Autodesk Inventor part; units mm, degrees
ref_plane "YZ Plane" through (0, 0, 0) normal (1, 0, 0) x (0, 1, 0)
ref_plane "XZ Plane" through (0, 0, 0) normal (0, 1, 0) x (-1, 0, 0)
ref_plane "XY Plane" through (0, 0, 0) normal (0, 0, 1) x (1, 0, 0)
sketch "Sketch1" plane through (0, 0, 0) normal (0, 1, 0) x (-1, 0, 0)
  line L0 (0, 0) -> (0, -6.35)
  line L1 (0, -6.35) -> (304.8, -6.35)
  line L2 (304.8, -6.35) -> (304.8, 0)
  line L3 (304.8, 0) -> (0, 0)
  dimension "d0" = 6.35
  dimension "d1" = 304.8
extrude "Extrusion1" add sketch "Sketch1" along normal blind 76.2
sketch "Sketch2" plane through (-304.8, 0, 0) normal (0, 0, 1) x (1, 0, 0)
  line L0 (273.812, 50.8) -> (96.012, 50.8)
  line L1 (96.012, 50.8) -> (96.012, 38.1)
  line L2 (96.012, 38.1) -> (273.812, 38.1)
  line L3 (273.812, 38.1) -> (273.812, 50.8)
  line L4 (96.012, 50.8) -> (35.1357, 42.2552)
  line L5 (35.1357, 42.2552) -> (36.5673, 32.0558)
  line L6 (36.5673, 32.0558) -> (97.4436, 40.6006)
  line L7 (97.4436, 40.6006) -> (96.012, 50.8)
  line L8 (0, 76.2) -> (304.8, 76.2)
  line L9 (304.8, 0) -> (304.8, 76.2)
  dimension "d4" = 177.8
  dimension "d5" = 12.7
  dimension "d24" = 25.4
  dimension "d25" = 30.988
sketch "Sketch3" plane through (-304.8, 0, 0) normal (0, 0, 1) x (1, 0, 0)
  point P0 (304.8, 0)
extrude "Extrusion2" cut sketch "Sketch2" against normal blind 6.35 contours L3 L2 L1 L6 L7 L0 | L7 L6 L1
sketch "Sketch4" plane through (-304.8, 0, 0) normal (0, 0, 1) x (1, 0, 0)
  point P0 (304.8, 0)
sketch "Sketch5" plane through (0, 0, -6.35) normal (0, 0, -1) x (-1, 0, 0)
  line L0 (0, 0) -> (0, 76.2)
  line L1 (0, 76.2) -> (6.35, 76.2)
  line L2 (6.35, 76.2) -> (6.35, 25.4)
  line L3 (6.35, 25.4) -> (0, 25.4)
  line L4 (0, 25.4) -> (0, 76.2)
  line L5 (0, 76.2) -> (304.8, 76.2)
  line L6 (0, 76.2) -> (6.35, 76.2)
  line L7 (6.35, 76.2) -> (6.35, 50.8)
  line L8 (6.35, 50.8) -> (0, 50.8)
  line L9 (0, 50.8) -> (0, 76.2)
  dimension "d8" = 6.35
  dimension "d9" = 50.8
  dimension "d11" = 25.4
extrude "Extrusion3" add sketch "Sketch5" along normal blind 25.4 contours L0 L8 L2 L3
sketch "Sketch6" plane through (-6.35, 25.4, -6.35) normal (-1, 0, 0) x (0, 0, 1)
  circle A0 centre (-11.9648, 20.32) radius 3.175
  circle A1 centre (-11.9648, 12.7) radius 1.5875
  line L0 (0, 0) -> (-25.4, 0)
  line L1 (-25.4, 25.4) -> (0, 25.4)
  point P0 (6.35, -25.4)
  dimension "d14" = 6.35
  dimension "d15" = 3.175
  dimension "d16" = 12.7
  dimension "d17" = 5.08
extrude "Extrusion4" cut sketch "Sketch6" against normal blind 6.35
sketch "Sketch7" plane through (0, 0, -6.35) normal (0, 0, -1) x (-1, 0, 0)
  line L0 (30.988, 38.1) -> (30.988, 50.8)
  line L1 (23.6557, 44.45) -> (27.3218, 50.8)
  line L2 (27.3218, 50.8) -> (34.6542, 50.8)
  line L3 (34.6542, 50.8) -> (38.3203, 44.45)
  line L4 (38.3203, 44.45) -> (34.6542, 38.1)
  line L5 (34.6542, 38.1) -> (27.3218, 38.1)
  line L6 (27.3218, 38.1) -> (23.6557, 44.45)
  line L7 (208.788, 50.8) -> (208.788, 38.1)
  line L8 (201.4557, 44.45) -> (205.1218, 50.8)
  line L9 (205.1218, 50.8) -> (212.4542, 50.8)
  line L10 (212.4542, 50.8) -> (216.1203, 44.45)
  line L11 (216.1203, 44.45) -> (212.4542, 38.1)
  line L12 (212.4542, 38.1) -> (205.1218, 38.1)
  line L13 (205.1218, 38.1) -> (201.4557, 44.45)
  point P0 (0, 0)
  point P1 (30.988, 44.45)
  point P2 (208.788, 44.45)
  dimension "d20" = 12.7
  dimension "d21" = 12.7
extrude "Extrusion5" cut sketch "Sketch7" against normal blind 6.35
properties part number "Plate add on"
Could you check a few things on this model? Use its own coordinates, in mm. A direction names the side the tool comes from. Round coordinates to 2 decimals unless told otherwise and drop trailing zeros. Write each loop counter-clockwise with the first axis right and the second up, starting at its lowest first coordinate (ties: lowest second). Pieces come first, ordered by that corner, then holes. Notation, with made-up numbers: (12.5, 46) -> (24.5, 46) arc R15 ccw to (24.5, 73) -> close; hole circle Ø4 at (-31, -20). An arc over 180 degrees is marked (long way). Use a Markdown table: item, result.
1. We'd pull the mould along X, two halves only. Please class faces 5 (the face through (-214.26, 47.67, -3.22)), 6 (the face through (0, 38, -12)), 7 (the face through (-6.35, 35, -19)): +X half, -X half, draft (parallel to the pull), parting line (faces both ways), or undercut.
Answer key:
| item | result |
|---|---|
| face 5 | undercut |
| face 6 | +X half |
| face 7 | -X half |
2. If we section it at A-A (z = -3.5): List the corners of the cut face in (x, y) for me.
Answer key:
| item | result |
|---|---|
| outline | (-304.8, 0) -> (0, 0) -> (0, 76.2) -> (-304.8, 76.2) -> close; hole (-216.12, 44.45) -> (-212.45, 38.1) -> (-27.32, 38.1) -> (-23.66, 44.45) -> (-27.32, 50.8) -> (-212.45, 50.8) -> close |
3. Which directions (+Z, -Z, +X, -X, +Y, -Y) give clear straight access to the entire face, cutting with the end or side of a thin tool? Please do faces 1 (the face through (-150, 76.2, -3)), 2 (the face through (-3, 25.4, -19)), 3 (the face through (-119, 50.8, -3)), 4 (the face through (-3, 50.8, -19)).
Answer key:
| item | result |
|---|---|
| face 1 | +Z, -Z, +X, -X, +Y |
| face 2 | -Z, +X, -X, -Y |
| face 3 | +Z, -Z |
| face 4 | -Z, +X, -X, +Y |
4. If we section it at B-B (x = -37): List the corners of the cut face in (y, z) for me.
Answer key:
| item | result |
|---|---|
| outline | (0, -6.35) -> (38.1, -6.35) -> (38.1, 0) -> (0, 0) -> close; (50.8, -6.35) -> (76.2, -6.35) -> (76.2, 0) -> (50.8, 0) -> close |
5. For pin 1 Ø5 at (x, z) = (-2, -22.5) entering from -Y; pin 2 Ø3 at (y, z) = (38.1, -18.31) entering from +X; pin 3 Ø3 at (x, y) = (-244, 47.5) entering from -Z; pin 4 Ø5 at (x, z) = (-4.5, -18) entering from +Y, each with a flat end and sliding along its axis, tell me the tip position at first contact or that it passes through.
Answer key:
| item | result |
|---|---|
| pin 1 | stops at y = 25.4 |
| pin 2 | passes through |
| pin 3 | stops at z = -6.35 |
| pin 4 | stops at y = 50.8 |
6. If we section it at C-C (x = -221.5): List the corners of the cut face in (y, z) for me.
Answer key:
| item | result |
|---|---|
| outline | (0, -6.35) -> (76.2, -6.35) -> (76.2, 0) -> (0, 0) -> close |
7. Please list where these lines run through material, in increasing order: probe 1 along Z at (x, y) = (-2, 38); probe 2 along Y at (x, z) = (-105, -1); probe 3 along Z at (x, y) = (-244, 22.5).
Answer key:
| item | result |
|---|---|
| probe 1 | z = -31.75 to -19.9, -16.73 to 0 |
| probe 2 | y = 0 to 38.1, 50.8 to 76.2 |
| probe 3 | z = -6.35 to 0 |
8. If we section it at D-D (y = 19): List the corners of the cut face in (x, z) for me, then the cut area to 3 significant figures.
Answer key:
| item | result |
|---|---|
| outline | (-304.8, -6.35) -> (0, -6.35) -> (0, 0) -> (-304.8, 0) -> close |
| area | 1,940 mm^2 |
